```python
from build123d import *

# Parameters (mm, degrees)
BOSS_EXTRUDE1_DEPTH  = 37.5
M6_CLEARANCE_HOLE1_D = 6.6
SKETCH7_W            = 9.4125
SKETCH7_H            = 13
CUT_EXTRUDE1_DEPTH   = 3.388423
CUT_EXTRUDE3_DEPTH   = 6.9125
MIRROR1_START        = 18.0875
MIRROR1_DEPTH        = 8.860423859
MIRROR1_2_DEPTH      = 6.9125
MIRROR1_START_2      = 6.9125
MIRROR1_3_OUTLINE_R  = 2.7
MIRROR1_3_DEPTH      = 11.175


# Read off the part's stored shape, not the designer's step: Mirror1
with BuildPart() as part:
    # Sketch1 → Boss-Extrude1 (new, symmetric)
    with BuildSketch(Plane(origin=(0, 0, 0), x_dir=(1, 0, 0), z_dir=(0, 1, 0))):
        with BuildLine():
            Line((-32.5, 0), (32.5, 0))
            Line((32.5, 0), (32.5, -10))
            Line((32.5, -10), (16.594252725, -10))
            ThreePointArc((16.594252725, -10), (15.639004066, -10.242871661), (14.915758236, -10.9125))
            Line((14.915758236, -10.9125), (6.148361062, -10.9125))
            ThreePointArc((6.148361062, -10.9125), (-6.35, -12.5), (6.148361062, -14.0875))
            Line((6.148361062, -14.0875), (14.915758236, -14.0875))
            ThreePointArc((14.915758236, -14.0875), (-0.794866801, -27.478924753), (-15, -12.5))
            Line((-15, -12.5), (-15, -11.958409852))
            ThreePointArc((-15, -11.958409852), (-15.448952846, -10.695772642), (-16.594252725, -10))
            Line((-16.594252725, -10), (-32.5, -10))
            Line((-32.5, -10), (-32.5, 0))
        make_face()
    extrude(amount=BOSS_EXTRUDE1_DEPTH, both=True)

    # M6 Clearance Hole1 (through all)
    with Locations(Plane(origin=(0, 0, 0), x_dir=(-1, 0, 0), z_dir=(0, 0, -1))):
        with Locations((25, -20), (-25, 20), (-25, -20), (25, 20)):
            Hole(M6_CLEARANCE_HOLE1_D / 2)

    # Sketch6 → Cut-Revolve1 (revolve, cut)
    with BuildSketch(Plane(origin=(10.532059649, 0, 0), x_dir=(0, 0, -1), z_dir=(1, 0, 0))):
        Polygon((0, 20), (-27.5, 20), (-27.5, 26.5), (-18.0875, 26.5), (-18.0875, 22.7), (0, 22.7), align=None)
    revolve(axis=Axis((10.532059649, 20, 0), (0, 0, 1)), mode=Mode.SUBTRACT)

    # Sketch7 → Cut-Extrude1 (cut)
    with BuildSketch(Plane(origin=(10.532059649, 0, 0), x_dir=(0, 0, -1), z_dir=(1, 0, 0))):
        with Locations((-22.79375, 20)):
            Rectangle(SKETCH7_W, SKETCH7_H)
    extrude(amount=CUT_EXTRUDE1_DEPTH, mode=Mode.SUBTRACT)

    # Sketch9 → Cut-Extrude3 (cut)
    with BuildSketch(Plane(origin=(0, 0, 0), x_dir=(-1, 0, 0), z_dir=(0, 0, -1))):
        Polygon((-6.282059649, 17.546261356), (-6.282059649, 22.453738644), (-10.532059649, 24.907477288), (-14.782059649, 22.453738644), (-14.782059649, 17.546261356), (-10.532059649, 15.092522712), align=None)
    extrude(amount=-CUT_EXTRUDE3_DEPTH, mode=Mode.SUBTRACT)

    # Mirror1 outline → Mirror1 (cut)
    with BuildSketch(Plane.XY.offset(MIRROR1_START)):
        with BuildLine():
            ThreePointArc((13.920482885, -14.453055979), (4.274858352, -18.240047747), (10.532059649, -26.5))
            Line((10.532059649, -26.5), (16, -26.5))
            Line((16, -26.5), (16, -15.723356181))
            Line((16, -15.723356181), (13.920482885, -14.453055979))
        make_face()
    extrude(amount=MIRROR1_DEPTH, mode=Mode.SUBTRACT)

    # Mirror1 2 outline → Mirror1 2 (cut)
    with BuildSketch(Plane.XY):
        Polygon((14.782059649, -22.453738644), (14.782059649, -17.546261356), (10.532059649, -15.092522712), (6.282059649, -17.546261356), (6.282059649, -22.453738644), (10.532059649, -24.907477288), align=None)
    extrude(amount=MIRROR1_2_DEPTH, mode=Mode.SUBTRACT)

    # Mirror1 3 outline → Mirror1 3 (cut)
    with BuildSketch(Plane.XY.offset(MIRROR1_START_2)):
        with Locations((10.532059649, -20)):
            Circle(MIRROR1_3_OUTLINE_R)
    extrude(amount=MIRROR1_3_DEPTH, mode=Mode.SUBTRACT)


solid = part.part
```
Could you check a few things on this model? Use its own coordinates, in mm. A direction names the side the tool comes from. Coordinates: 2 decimals unless noted, no trailing zeros. Write each loop counter-clockwise with the first axis right and the second up, starting at its lowest first coordinate (ties: lowest second). Pieces come first, ordered by that corner, then holes. Notation, with made-up numbers: M 55,33 L 77,33 A21 ccw 77,65 Z; hole C 66.25,38 d4. An arc over 180 degrees is marked long. Answer as CSV lines item,"result". Start each with the question number.
1) Please list where these lines run through material, in increasing order: line 1 (Y direction, x = 25, z = 4); line 2 (X direction, y = -23, z = 3); line 3 (X direction, y = -20, z = 16.5). Write a range as from..to.
2) I want a section at A-A, the plane x = 0. Please give me the cut outline in (y, z), and give its area (3 significant figures).
3) I want a section at D-D, the plane z = 9. Please give me the cut outline in (x, y), and give its area (3 significant figures).
4) We'd pull the mould along X, two halves only. Please class faces 6 (the cylindrical face through (-21.95, 18.74, 5.07)), 7 (the cylindrical face through (-0.476, 0.525, 27.492)), 8 (the cylindrical face through (-15.44, 0.52, 10.71)), 9 (the flat face through (10, 1, 14.088)): +X half, -X half, draft (parallel to the pull), parting line (faces both ways), or undercut.
5) For faces 1 (the flat face through (11, 1, 10.912)), 2 (the flat face through (-24, 1, 10)), 3 (the cylindrical face through (4.07, -20.71, 21.47)), 4 (the flat face through (8.44, 16.3, 3.41)), 5 (the flat face through (0, -37.5, 4)), which set-ups out of +Z, -Z, +X, -X, +Y, -Y let a thin tool reach every point of the face, with its end or its side?
6) I want a section at B-B, the plane z = 2.5. Please give me the cut outline in (x, y), and give its area (3 significant figures).
7) I want a section at C-C, the plane x = 25. Please give me the cut outline in (y, z).
8) For P1, Ø8.5, axis at x = -25, y = -20, coming from the +Z side; P2, Ø4, axis at x = 12.5, y = 21.5, coming from the -Z side; P3, Ø11, axis at x = 9.5, y = 22.5, coming from the +Z side; P4, Ø7, axis at x = 11.5, y = -14.5, coming from the +Z side, each with a flat end and sliding along its axis, tell me the tip position at first contact or that it passes through.
Data:
1,line 1,"y = -37.5..-23.3, -16.7..16.7, 23.3..37.5"
1,line 2,"x = -32.5..-26.37, -23.63..7.23, 13.84..23.63, 26.37..32.5"
1,line 3,"x = -14.46..-4.93, 4.93..7.83, 13.23..14.46"
2,outline,"M -37.5,0 L 37.5,0 L 37.5,6.15 L -37.5,6.15 Z; M -37.5,18.85 L 37.5,18.85 L 37.5,27.5 L -37.5,27.5 Z"
2,area,"1,110 mm^2"
3,outline,"M -32.5,-37.5 L -5.3,-37.5 L -5.3,37.5 L -32.5,37.5 Z; M 5.3,-37.5 L 32.5,-37.5 L 32.5,37.5 L 5.3,37.5 Z; hole C -25,-20 d6.6; hole C -25,20 d6.6; hole C 10.53,-20 d5.4; hole C 10.53,20 d5.4; hole C 25,-20 d6.6; hole C 25,20 d6.6"
3,area,"3,900 mm^2"
4,face 6,"undercut"
4,face 7,"parting line"
4,face 8,"-X half"
4,face 9,"draft"
5,face 1,"+X, +Y, -Y"
5,face 2,"+Z, -X, +Y, -Y"
5,face 3,"+Z"
5,face 4,"-Z"
5,face 5,"+Z, -Z, +X, -X, -Y"
6,outline,"M -32.5,-37.5 L 32.5,-37.5 L 32.5,37.5 L -32.5,37.5 Z; hole C -25,-20 d6.6; hole C -25,20 d6.6; hole M 6.28,-22.45 L 10.53,-24.91 L 14.78,-22.45 L 14.78,-17.55 L 10.53,-15.09 L 6.28,-17.55 Z; hole M 6.28,17.55 L 10.53,15.09 L 14.78,17.55 L 14.78,22.45 L 10.53,24.91 L 6.28,22.45 Z; hole C 25,-20 d6.6; hole C 25,20 d6.6"
6,area,"4,610 mm^2"
7,outline,"M -37.5,0 L -23.3,0 L -23.3,10 L -37.5,10 Z; M -16.7,0 L 16.7,0 L 16.7,10 L -16.7,10 Z; M 23.3,0 L 37.5,0 L 37.5,10 L 23.3,10 Z"
8,P1,"stops at z = 10"
8,P2,"stops at z = 0"
8,P3,"stops at z = 26.96"
8,P4,"stops at z = 25.17"
